Geometry check sheet. Reference: the model listing, model coordinates, mm. A direction names the side the tool comes from. Give positions to 0.01 mm unless a question says otherwise; leave off trailing zeros. Loops run counter-clockwise (first coordinate to the right, second up) from the corner with the lowest first, then second, coordinate; pieces in that order, holes last. Notation, with made-up numbers: (-18.5, 17.25) -> (-8.5, 17.25) arc R18 ccw to (-8.5, 42.25) -> close; hole circle Ø10 at (-1, 54). An arc over 180 degrees is marked (long way). One line per question, with ' | ' between items.
from build123d import *

# Parameters (mm, degrees)
BOSS_EXTRUDE1_DEPTH = 36
SKETCH2_R           = 2
CUT_EXTRUDE1_DEPTH  = 29
SKETCH3_R           = 2
BOSS_EXTRUDE2_DEPTH = 10


with BuildPart() as part:
    # Sketch1 → Boss-Extrude1 (new body)
    with BuildSketch(Plane.XY):
        Polygon((2.598076211, -1.5), (2.598076211, 1.5), (0, 3), (-2.598076211, 1.5), (-2.598076211, -1.5), (0, -3), align=None)
    extrude(amount=-BOSS_EXTRUDE1_DEPTH)

    # Sketch2 → Cut-Extrude1 (cut)
    with BuildSketch(Plane.XY):
        Circle(SKETCH2_R)
    extrude(amount=-CUT_EXTRUDE1_DEPTH, mode=Mode.SUBTRACT)

    # Sketch3 → Boss-Extrude2 (add)
    with BuildSketch(Plane(origin=(0, 0, -36), x_dir=(-1, 0, 0), z_dir=(0, 0, -1))):
        Circle(SKETCH3_R)
    extrude(amount=BOSS_EXTRUDE2_DEPTH)


solid = part.part
Item 1: Sectioned sample at B-B (y = -0.6). Record the cut outline in (x, z).
Result:
outline: (-2.6, -36) -> (-1.91, -36) -> (-1.91, -46) -> (1.91, -46) -> (1.91, -36) -> (2.6, -36) -> (2.6, 0) -> (1.91, 0) -> (1.91, -29) -> (-1.91, -29) -> (-1.91, 0) -> (-2.6, 0) -> close
Item 2: Depth check by flat-ended pin: pin 1 Ø3 at (x, z) = (2, -39) entering from -Y; pin 2 Ø2 at (x, y) = (0.5, -0.5) entering from +Z; pin 3 Ø2 at (y, z) = (-1.5, -39.5) entering from +X. Enter the tip coordinate at first touch or a pass-through.
Result:
pin 1: y = -1.94 | pin 2: z = -29 | pin 3: x = 1.94
Item 3: Release check for a two-part mould opening along Y. For faces 1 (the face through (0, -2, -14)), 2 (the face through (1.28, -2.26, -17.75)), 3 (the face through (1.32, 2.24, -17.75)), 4 (the face through (0, 0, -29)) record: pulls with the +Y half, pulls with the -Y half, needs draft (parallel to the pull), parting line crosses it, or undercut.
Result:
face 1: undercut | face 2: pulls with the -Y half | face 3: pulls with the +Y half | face 4: undercut
Item 4: Scan lines: probe 1 along Y at (x, z) = (0, -20.25); probe 2 along Z at (x, y) = (0.8, 1.35); probe 3 along X at (y, z) = (-1.8, -16). Record each from-to range of solid material in increasing order.
Result:
probe 1: -3 to -2, 2 to 3 | probe 2: -46 to -29 | probe 3: -2.08 to -0.87, 0.87 to 2.08
Item 5: Sectioned sample at C-C (z = -35.5). Record the cut outline in (x, y), plus the area to 3 significant figures.
Result:
outline: (-2.6, -1.5) -> (0, -3) -> (2.6, -1.5) -> (2.6, 1.5) -> (0, 3) -> (-2.6, 1.5) -> close | area: 23.4 mm2
Item 6: Sectioned sample at A-A (z = -20). Record the cut outline in (x, y).
Result:
outline: (-2.6, -1.5) -> (0, -3) -> (2.6, -1.5) -> (2.6, 1.5) -> (0, 3) -> (-2.6, 1.5) -> close; hole circle Ø4 at (0, 0)
Item 7: Set-up check for faces 5 (the face through (-1.32, -2.24, -17.75)), 6 (the face through (-1, 2, -36)): record each of +Z, -Z, +X, -X, +Y, -Y from which the full face is reachable in a straight line by a thin tool's end or side.
Result:
face 5: +Z, -Z, -X, -Y | face 6: -Z
Item 8: Sectioned sample at D-D (x = -0.7). Record the cut outline in (y, z), plus the area to 3 significant figures.
Result:
outline: (-2.6, -36) -> (-1.87, -36) -> (-1.87, -46) -> (1.87, -46) -> (1.87, -36) -> (2.6, -36) -> (2.6, 0) -> (1.87, 0) -> (1.87, -29) -> (-1.87, -29) -> (-1.87, 0) -> (-2.6, 0) -> close | area: 116 mm2
